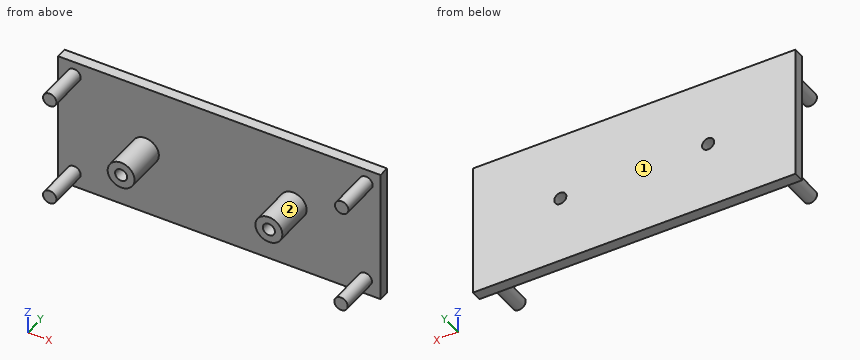
```python
from build123d import *

# Parameters (mm, degrees)
F0_R     = 2.25
F1_DEPTH = 4
F2_R     = 5
F2_R_2   = 2.25
F3_DEPTH = 15
F4_R     = 2.5
F5_DEPTH = 15


with BuildPart() as f1:
    # F0 (on Front) → F1 (new body)
    with BuildSketch(Plane.XZ):
        Polygon((-60, -25), (0, -25), (60, -25), (60, 25), (-60, 25), align=None)
        with Locations((-27.5, 0)):
            Circle(F0_R, mode=Mode.SUBTRACT)
        with Locations((27.5, 0)):
            Circle(F0_R, mode=Mode.SUBTRACT)
    extrude(amount=F1_DEPTH)

    # F2 (on face) → F3 (join)
    with BuildSketch(Plane.XZ.offset(4)):
        with Locations((-27.5, 0)):
            Circle(F2_R)
        with Locations((-27.5, 0)):
            Circle(F2_R_2, mode=Mode.SUBTRACT)
        with Locations((27.5, 0)):
            Circle(F2_R)
        with Locations((27.5, 0)):
            Circle(F2_R_2, mode=Mode.SUBTRACT)
    extrude(amount=F3_DEPTH)

    # F4 (on face) → F5 (join)
    with BuildSketch(Plane.XZ.offset(4)):
        with Locations((-54.076705, 19.686049)):
            Circle(F4_R)
        with Locations((-54.076705, -19.433273)):
            Circle(F4_R)
        with Locations((54.332387, -19.177591)):
            Circle(F4_R)
        with Locations((54.588076, 19.686049)):
            Circle(F4_R)
    extrude(amount=F5_DEPTH)


solid = f1.part
```
Input: part model. Units: mm. Frame: model coordinates. Face numbers are marked on the shaded views. Coordinates: 2 decimals unless noted, no trailing zeros. Loops run counter-clockwise (first coordinate to the right, second up) from the corner with the lowest first, then second, coordinate; pieces in that order, holes last. Notation, with made-up numbers: (85.25, 54.25) - (132.25, 54.25) arc R15 cw to (132.25, 80.25) - close; hole circle Ø8 at (76, -26.75). An arc over 180 degrees is marked (long way). Answer in a Markdown table with one row per item.
(1) Mould query, pull axis X, two halves, no side actions, for the marked faces 1 and 2. Classes: pulls with the +X half, pulls with the -X half, needs draft (parallel to the pull), parting line crosses it, or undercut.
Model answer:
| item | result |
|---|---|
| face 1 | needs draft |
| face 2 | undercut |
(2) Cut plane D-D on x = 4.5. Output: boundary loops of the cut face in (y, z), plus the area to 3 significant figures.
Model answer:
| item | result |
|---|---|
| outline | (-4, -25) - (0, -25) - (0, 25) - (-4, 25) - close |
| area | 200 mm² |
(3) Cut plane A-A on z = 0. Output: boundary loops of the cut face in (x, y).
Model answer:
| item | result |
|---|---|
| outline | (-60, -4) - (-32.5, -4) - (-32.5, -19) - (-29.75, -19) - (-29.75, 0) - (-60, 0) - close; (-25.25, -19) - (-22.5, -19) - (-22.5, -4) - (22.5, -4) - (22.5, -19) - (25.25, -19) - (25.25, 0) - (-25.25, 0) - close; (29.75, -19) - (32.5, -19) - (32.5, -4) - (60, -4) - (60, 0) - (29.75, 0) - close |
(4) Cut plane B-B on y = -6.75. Output: boundary loops of the cut face in (x, z), plus the area to 3 significant figures.
Model answer:
| item | result |
|---|---|
| outline | circle Ø5 at (-54.08, -19.43); circle Ø5 at (-54.08, 19.69); circle Ø10 at (-27.5, 0); circle Ø10 at (27.5, 0); circle Ø5 at (54.33, -19.18); circle Ø5 at (54.59, 19.69); hole circle Ø4.5 at (-27.5, 0); hole circle Ø4.5 at (27.5, 0) |
| area | 204 mm² |
(5) Pin query (flat end, axial travel): P1, Ø3, axis at y = -14.5, z = 17.5, coming from the -X side; P2, Ø2.5, axis at x = -27.5, z = 0, coming from the +Y side. Return the tip coordinate at first contact, or that it passes through.
Model answer:
| item | result |
|---|---|
| P1 | stops at x = -56.48 |
| P2 | passes through |
(6) Cut plane C-C on x = -27.5. Output: boundary loops of the cut face in (y, z), plus the area to 4 significant figures.
Model answer:
| item | result |
|---|---|
| outline | (-19, -5) - (-4, -5) - (-4, -25) - (0, -25) - (0, -2.25) - (-19, -2.25) - close; (-19, 2.25) - (0, 2.25) - (0, 25) - (-4, 25) - (-4, 5) - (-19, 5) - close |
| area | 264.5 mm² |
(7) Material intervals for L1, parallel to Z at x = -27.5, y = -9.5; L2, parallel to Y at x = 10.5, z = 6.5; L3, parallel to Z at x = 27.5, y = -3.75, sorted ascending. Write a range as from..to.
Model answer:
| item | result |
|---|---|
| L1 | z = -5..-2.25, 2.25..5 |
| L2 | y = -4..0 |
| L3 | z = -25..-2.25, 2.25..25 |
